```python
from build123d import *

# Parameters (mm, degrees)
SKETCH8_R          = 4
CUT_EXTRUDE1_DEPTH = 121
SKETCH8_9_R        = 10
CUT_EXTRUDE2_DEPTH = 90


with BuildPart() as part:
    # Sketch6 → Revolve1 (revolve)
    with BuildSketch(Plane.YZ, mode=Mode.PRIVATE) as revolve1_sk:
        Polygon((0, 0), (-100, 0), (-100, 25), (-50, 100), (0, 100), align=None)
    revolve(revolve1_sk.sketch.rotate(Axis((0, 0, 100), (0, 0, -1)), 270), axis=Axis((0, 0, 100), (0, 0, -1)))

    # Sketch7 → Cut-Revolve1 (revolve, cut)
    with BuildSketch(Plane(origin=(0, 0, 0), x_dir=(-1, 0, 0), z_dir=(0, 1, 0)), mode=Mode.PRIVATE) as cut_revolve1_sk:
        Polygon((0, 25), (-45, 25), (-60, 25), (-60, 60), (-45, 60), (-45, 100), (0, 100), align=None)
    revolve(cut_revolve1_sk.sketch.rotate(Axis((0, 0, 25), (0, 0, 1)), 180), axis=Axis((0, 0, 25), (0, 0, 1)), mode=Mode.SUBTRACT)

    # Sketch8 → Cut-Extrude1 (cut)
    with BuildSketch(Plane.XY.offset(100)):
        with Locations(Location((-60.710678119, 60.710678119, 0), (0, 0, 133.397835017))):
            Circle(SKETCH8_R)
        with Locations(Location((60.710678119, 60.710678119, 0), (0, 0, 45))):
            Circle(SKETCH8_R)
        with Locations(Location((60.710678119, -60.710678119, 0), (0, 0, 315))):
            Circle(SKETCH8_R)
        with Locations(Location((-60.710678119, -60.710678119, 0), (0, 0, 225))):
            Circle(SKETCH8_R)
    extrude(amount=-CUT_EXTRUDE1_DEPTH, mode=Mode.SUBTRACT)

    # Sketch8_9 → Cut-Extrude2 (cut)
    with BuildSketch(Plane.XY.offset(100)):
        with Locations((-60.710678119, 60.710678119)):
            Circle(SKETCH8_9_R)
        with Locations((60.710678119, 60.710678119)):
            Circle(SKETCH8_9_R)
        with Locations((60.710678119, -60.710678119)):
            Circle(SKETCH8_9_R)
        with Locations((-60.710678119, -60.710678119)):
            Circle(SKETCH8_9_R)
    extrude(amount=-CUT_EXTRUDE2_DEPTH, mode=Mode.SUBTRACT)


solid = part.part
```
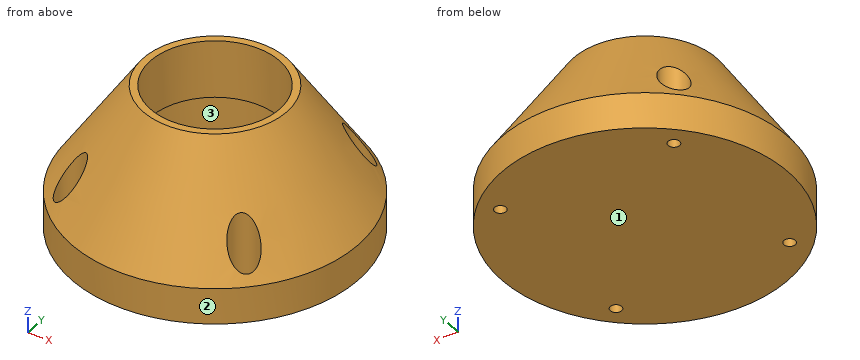
Can you work these out from the model? Positions are in its coordinate system, mm. Face numbers are marked on the shaded views. Round coordinates to 2 decimals unless told otherwise and drop trailing zeros. Loops run counter-clockwise (first coordinate to the right, second up) from the corner with the lowest first, then second, coordinate; pieces in that order, holes last. Notation, with made-up numbers: (-6.75, 26.5) -> (44.25, 26.5) arc R9 cw to (44.25, 38.5) -> close; hole circle Ø9 at (85, -12). An arc over 180 degrees is marked (long way). One line per item, written item: value. Start each with the question number.
1. If we mould it in two halves opening along Y, with no side actions, what happens to the marked faces 1, 2 and 3? For each: pulls with the +Y half, pulls with the -Y half, needs draft (parallel to the pull), parting line crosses it, or undercut.
2. For pin 1 (3 mm diameter, centred on x = -22, z = 30.5, fed in from +Y); pin 2 (1.5 mm diameter, centred on x = 21, z = 40.5, fed in from -Y); pin 3 (4 mm diameter, centred on x = -13.5, y = 8, fed in from +Z); pin 4 (12 mm diameter, centred on x = 11.5, y = 7, fed in from -Z), each with a flat end and sliding along its axis, tell me the tip position at first contact or that it passes through.
3. If I drill on probe 1 along Z at (x, y) = (44, 16.5); probe 2 along X at (y, z) = (59, 20); probe 3 along Y at (x, z) = (-61, 23), over which ranges is the centre line in solid material (lowest first)?
4. If we section it at C-C, the plane z = 45: Write out the boundary of the cut face in (x, y).
5. If we section it at A-A, the plane x = 0: Write out the boundary of the cut face in (y, z), then the cut area to 3 significant figures.
6. If we section it at D-D, the plane z = 18.5: Write out the boundary of the cut face in (x, y).
Calculated:
1. face 1: needs draft
1. face 2: parting line crosses it
1. face 3: undercut
2. pin 1: stops at y = 94.87
2. pin 2: stops at y = -87.72
2. pin 3: stops at z = 25
2. pin 4: stops at z = 0
3. probe 1: z = 0 to 25, 60 to 100
3. probe 2: x = -80.74 to -70.56, -50.86 to 50.86, 70.56 to 80.74
3. probe 3: y = -79.24 to -70.71, -50.71 to 50.71, 70.71 to 79.24
4. outline: (-67.94, -53.8) arc R10 cw (long way) to (-53.8, -67.94) arc R86.67 ccw to (53.8, -67.94) arc R10 cw (long way) to (67.94, -53.8) arc R86.67 ccw to (67.94, 53.8) arc R10 cw (long way) to (53.8, 67.94) arc R86.67 ccw to (-53.8, 67.94) arc R10 cw (long way) to (-67.94, 53.8) arc R86.67 ccw to start; hole circle Ø120 at (0, 0)
5. outline: (-100, 0) -> (100, 0) -> (100, 25) -> (50, 100) -> (45, 100) -> (45, 60) -> (60, 60) -> (60, 25) -> (-60, 25) -> (-60, 60) -> (-45, 60) -> (-45, 100) -> (-50, 100) -> (-100, 25) -> close
5. area: 8,450 mm²
6. outline: circle Ø200 at (0, 0); hole circle Ø20 at (-60.71, -60.71); hole circle Ø20 at (-60.71, 60.71); hole circle Ø20 at (60.71, -60.71); hole circle Ø20 at (60.71, 60.71)
